Design review of the part built by this model. Coordinates are the model's own, in mm. Face numbers are marked on the shaded views. A direction names the side the tool comes from. Coordinates: 2 decimals unless noted, no trailing zeros. Loops run counter-clockwise (first coordinate to the right, second up) from the corner with the lowest first, then second, coordinate; pieces in that order, holes last. Notation, with made-up numbers: (7.25, -7.75) -> (40.25, -7.75) arc R21 ccw to (40.25, 22.25) -> close; hole circle Ø11 at (65.25, 18.5). An arc over 180 degrees is marked (long way). Use a Markdown table: item, result. Add a question column.
Q1. Draft analysis for pull direction X (two halves, no side actions). For the marked faces 1, 2 and 3, state which applies: pulls with the +X half, pulls with the -X half, needs draft (parallel to the pull), parting line crosses it, or undercut.
Q2. Take a section at C-C on z = 4.5. Write out the cut boundary in (x, y), plus the area to 3 significant figures.
Q3. Take a section at A-A on x = 52.5. Write out the cut boundary in (y, z), plus the area to 3 significant figures.
Q4. Clearance check with flat-ended pins moving along their axes: pin 1 Ø5.5 at (x, z) = (26.5, -10) entering from +Y; pin 2 Ø2 at (y, z) = (3, 16) entering from -X; pin 3 Ø4.5 at (y, z) = (2, 15) entering from +X; pin 4 Ø4 at (x, z) = (7.5, -7.5) entering from -Y. State where each tip first meets the part, or that it passes through.
Q5. For the marked faces 4, 5 and 6, list the 3-axis set-ups (+Z, -Z, +X, -X, +Y, -Y) from which the entire face can be reached by the end or side of a thin tool; tool diameter is ignored.
Q6. For probe 1 along X at (y, z) = (10.5, 15.2); probe 2 along Z at (x, y) = (38, 12.5); probe 3 along X at (y, z) = (13.75, 1), list the stretches that pass through material, from the lowest coordinate up.
Q7. Take a section at B-B on z = -7.5. Write out the cut boundary in (x, y), plus the area to 3 significant figures.
Q8. Take a section at D-D on x = 26.5. Write out the cut boundary in (y, z).
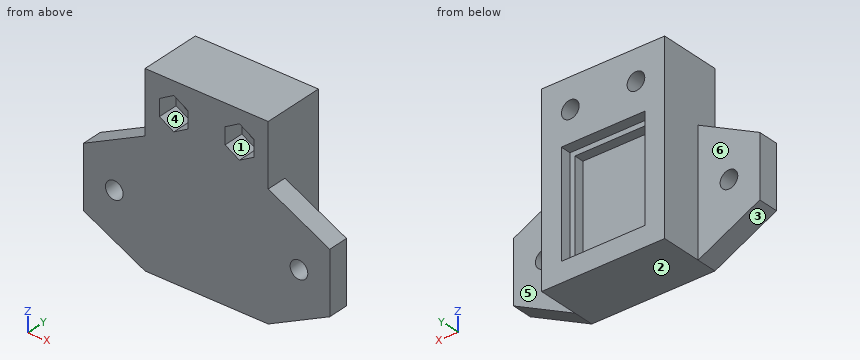
from build123d import *

# Parameters (mm, degrees)
SKETCH1_W                = 30
SKETCH1_H                = 30
BOSS_EXTRUDE1_DEPTH      = 5
M4_CLEARANCE_HOLE1_D     = 4.3
M4_CLEARANCE_HOLE1_DEPTH = 5
SKETCH13_W               = 30
SKETCH13_H               = 45
BOSS_EXTRUDE7_DEPTH      = 15
SKETCH14_W               = 20.4
SKETCH14_H               = 25.4
CUT_EXTRUDE2_DEPTH       = 5
BOSS_EXTRUDE8_REACH      = 19.6
BOSS_EXTRUDE8_START      = -2.6
SKETCH15_W               = 20.4
SKETCH15_H               = 25.4
SKETCH15_W_2             = 18
SKETCH15_H_2             = 23
M4_CLEARANCE_HOLE2_D     = 4.3
M4_CLEARANCE_HOLE2_DEPTH = 15
CUT_EXTRUDE1_DEPTH       = 5


with BuildPart() as part:
    # Sketch1 → Boss-Extrude1 (new body)
    with BuildSketch(Plane(origin=(0, 0, 0), x_dir=(1, 0, 0), z_dir=(0, 1, 0))):
        Polygon((15, 22.5), (15, -7.5), (0, 0), (0, 15), align=None)
        with Locations((30, 7.5)):
            Rectangle(SKETCH1_W, SKETCH1_H)
        Polygon((45, -7.5), (45, 22.5), (60, 15), (60, 0), align=None)
    extrude(amount=BOSS_EXTRUDE1_DEPTH)

    # M4 Clearance Hole1
    with Locations(Plane(origin=(0, 0, 0), x_dir=(-1, 0, 0), z_dir=(0, -1, 0))):
        with Locations((-7.5, 7.5), (-52.5, 7.5)):
            Hole(M4_CLEARANCE_HOLE1_D / 2, depth=M4_CLEARANCE_HOLE1_DEPTH)

    # Sketch13 → Boss-Extrude7 (add)
    with BuildSketch(Plane(origin=(0, 0, 0), x_dir=(1, 0, 0), z_dir=(0, 1, 0))):
        with Locations((30, 0)):
            Rectangle(SKETCH13_W, SKETCH13_H)
    extrude(amount=BOSS_EXTRUDE7_DEPTH)

    # Sketch14 → Cut-Extrude2 (cut)
    with BuildSketch(Plane(origin=(0, 15, 0), x_dir=(1, 0, 0), z_dir=(0, 1, 0))):
        with Locations((30, 5)):
            Rectangle(SKETCH14_W, SKETCH14_H)
    extrude(amount=-CUT_EXTRUDE2_DEPTH, mode=Mode.SUBTRACT)

    # Sketch15 → Boss-Extrude8 (add, up to next)
    with BuildSketch(Plane(origin=(0, 15, 0), x_dir=(1, 0, 0), z_dir=(0, 1, 0)).offset(BOSS_EXTRUDE8_START), mode=Mode.PRIVATE) as boss_extrude8_sk1:
        with Locations((30, 5)):
            Rectangle(SKETCH15_W, SKETCH15_H)
        with Locations((30, 5)):
            Rectangle(SKETCH15_W_2, SKETCH15_H_2, mode=Mode.SUBTRACT)
    boss_extrude8_tool1 = extrude(boss_extrude8_sk1.sketch, amount=-BOSS_EXTRUDE8_REACH, mode=Mode.PRIVATE) - part.part
    add(boss_extrude8_tool1.solids().sort_by_distance((39.874221, 12.4, -5))[0])

    # M4 Clearance Hole2
    with Locations(Plane(origin=(0, 15, 0), x_dir=(1, 0, 0), z_dir=(0, 1, 0))):
        with Locations((22, -15.2), (38, -15.2)):
            Hole(M4_CLEARANCE_HOLE2_D / 2, depth=M4_CLEARANCE_HOLE2_DEPTH)

    # Sketch11 → Cut-Extrude1 (cut)
    with BuildSketch(Plane(origin=(0, 0, 0), x_dir=(-1, 0, 0), z_dir=(0, 1, 0))):
        Polygon((-22, 19.241451884), (-25.5, 17.220725942), (-25.5, 13.179274058), (-22, 11.158548116), (-18.5, 13.179274058), (-18.5, 17.220725942), align=None)
    cut_extrude1 = extrude(amount=CUT_EXTRUDE1_DEPTH, mode=Mode.SUBTRACT)

    # Mirror1: Cut-Extrude1 across plane
    add(cut_extrude1.mirror(Plane(origin=(30, 0, 0), x_dir=(0, 0, 1), z_dir=(1, 0, 0))), mode=Mode.SUBTRACT)


solid = part.part
Answer list:
| question | item | result |
|---|---|---|
| 1 | face 1 | undercut |
| 1 | face 2 | needs draft |
| 1 | face 3 | pulls with the -X half |
| 2 | outline | (9, 0) -> (51, 0) -> (51, 5) -> (45, 5) -> (45, 15) -> (40.2, 15) -> (40.2, 12.4) -> (39, 12.4) -> (39, 10) -> (21, 10) -> (21, 12.4) -> (19.8, 12.4) -> (19.8, 15) -> (15, 15) -> (15, 5) -> (9, 5) -> close |
| 2 | area | 414 mm² |
| 3 | outline | (0, -18.75) -> (5, -18.75) -> (5, -9.65) -> (0, -9.65) -> close; (0, -5.35) -> (5, -5.35) -> (5, 3.75) -> (0, 3.75) -> close |
| 3 | area | 91.0 mm² |
| 4 | pin 1 | y = 10 |
| 4 | pin 2 | x = 15 |
| 4 | pin 3 | x = 45 |
| 4 | pin 4 | through |
| 5 | face 4 | -Y |
| 5 | face 5 | +Z, -Z, +X, +Y |
| 5 | face 6 | +Z, -Z, -X, +Y |
| 6 | probe 1 | 15 to 19.85, 24.15 to 35.85, 40.15 to 45 |
| 6 | probe 2 | -22.5 to -17.7, 7.7 to 13.05, 17.35 to 22.5 |
| 6 | probe 3 | 15 to 19.8, 40.2 to 45 |
| 7 | outline | (0, 0) -> (5.35, 0) -> (5.35, 5) -> (0, 5) -> close; (9.65, 0) -> (50.35, 0) -> (50.35, 5) -> (45, 5) -> (45, 15) -> (40.2, 15) -> (40.2, 12.4) -> (39, 12.4) -> (39, 10) -> (21, 10) -> (21, 12.4) -> (19.8, 12.4) -> (19.8, 15) -> (15, 15) -> (15, 5) -> (9.65, 5) -> close; (54.65, 0) -> (60, 0) -> (60, 5) -> (54.65, 5) -> close |
| 7 | area | 461 mm² |
| 8 | outline | (0, -22.5) -> (15, -22.5) -> (15, -17.7) -> (12.4, -17.7) -> (12.4, -16.5) -> (10, -16.5) -> (10, 6.5) -> (12.4, 6.5) -> (12.4, 7.7) -> (15, 7.7) -> (15, 22.5) -> (0, 22.5) -> close |
